Input: dimensioned drawing with shaded views. Units: mm. Origin: part minimum x, y, z. A direction names the side the tool comes from. Round coordinates to 2 decimals unless told otherwise and drop trailing zeros. Loops run counter-clockwise (first coordinate to the right, second up) from the corner with the lowest first, then second, coordinate; pieces in that order, holes last. Notation, with made-up numbers: M 80.5,8.5 L 110.5,8.5 A19 cw 110.5,44.5 Z; hole C -10,-18 d6. An arc over 180 degrees is marked long. Return JSON: item names as keys, results as strings.
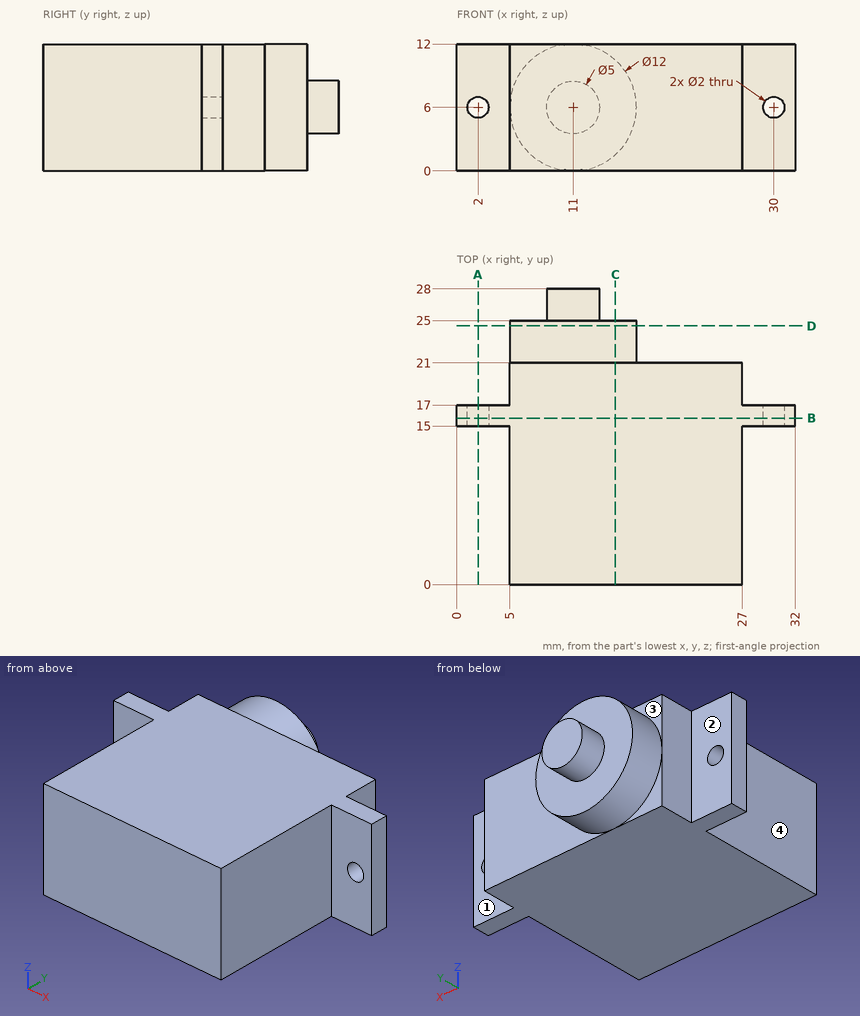
Q1. Material intervals for L1, parallel to X at y = 15.6, z = 6; L2, parallel to Z at x = 30, y = 15.9; L3, parallel to Y at x = 22.5, z = 7.25, sorted ascending.
Determined:
{"L1": "x = 0 to 1, 3 to 29, 31 to 32", "L2": "z = 0 to 5, 7 to 12", "L3": "y = 0 to 21"}
Q2. Section query D-D (y = 24.5). Output: boundary loops of the cut face in (x, z).
Determined:
{"outline": "C 11,6 d12"}
Q3. Section query A-A (x = 2). Output: boundary loops of the cut face in (y, z).
Determined:
{"outline": "M 15,0 L 17,0 L 17,5 L 15,5 Z; M 15,7 L 17,7 L 17,12 L 15,12 Z"}
Q4. Section query C-C (x = 15). Output: boundary loops of the cut face in (y, z), plus the area to 3 significant figures.
Determined:
{"outline": "M 0,0 L 21,0 L 21,1.53 L 25,1.53 L 25,10.47 L 21,10.47 L 21,12 L 0,12 Z", "area": "288 mm^2"}
Q5. Reachability of the marked faces 1, 2, 3 and 4 from +Z, -Z, +X, -X, +Y, -Y: full face, straight path, thin tool, end or side. Return the list, or none.
Determined:
{"face 1": "+Z, -Z, +X, +Y", "face 2": "+Z, -Z, -X, +Y", "face 3": "+Z, -X, +Y", "face 4": "+Z, -Z, -X, -Y"}
Q6. Pin query (flat end, axial travel): pin 1 (1.2 mm diameter, centred on x = 30, z = 6, fed in from +Y); pin 2 (2.5 mm diameter, centred on x = 3, z = 7.5, fed in from +Y); pin 3 (5.5 mm diameter, centred on x = 30, z = 9, fed in from -Y); pin 4 (3 mm diameter, centred on x = 7, z = 9.5, fed in from +Y). Return the tip coordinate at first contact, or that it passes through.
Determined:
{"pin 1": "passes through", "pin 2": "stops at y = 17", "pin 3": "stops at y = 15", "pin 4": "stops at y = 25"}
Q7. Section query B-B (y = 15.75). Output: boundary loops of the cut face in (x, z).
Determined:
{"outline": "M 0,0 L 32,0 L 32,12 L 0,12 Z; hole C 2,6 d2; hole C 30,6 d2"}
